```python
from build123d import *

# Parameters (mm, degrees)
SKETCH1_R           = 38.1
BOSS_EXTRUDE1_DEPTH = 4.826
SKETCH2_R           = 38.1
BOSS_EXTRUDE2_DEPTH = 3.302
BOSS_EXTRUDE2_DRAFT = -70
SKETCH3_R           = 47.172170439
BOSS_EXTRUDE3_DEPTH = 3.81
SKETCH4_R           = 46.472170439
CUT_EXTRUDE1_DEPTH  = 0.2
SKETCH6_R           = 34.772170439
SKETCH6_R_2         = 12.7
CUT_EXTRUDE2_DEPTH  = 2.7
SKETCH8_R           = 12.7
BOSS_EXTRUDE4_DEPTH = 50.8
SKETCH10_R          = 7.35
CUT_EXTRUDE5_DEPTH  = 3
SKETCH13_R          = 6.4
CUT_EXTRUDE9_DEPTH  = 92.577748235
SKETCH15_R          = 37.5
BOSS_EXTRUDE6_DEPTH = 8
CUT_EXTRUDE10_REACH = 99.233
SKETCH16_R          = 2
SKETCH16_R_2        = 5.35
SKETCH17_R          = 20.71
SKETCH17_R_2        = 19.21
CUT_EXTRUDE11_DEPTH = 3


with BuildPart() as part:
    # Sketch1 → Boss-Extrude1 (new body)
    with BuildSketch(Plane(origin=(0, 0, 0), x_dir=(1, 0, 0), z_dir=(0, 1, 0))):
        with Locations(Location((0, 0, 0), (0, 0, 270))):
            Circle(SKETCH1_R)
    extrude(amount=BOSS_EXTRUDE1_DEPTH)


with BuildPart() as boss_extrude2_tool:
    # Sketch2 → Boss-Extrude2 (with draft: the straight prism first)
    with BuildSketch(Plane(origin=(0, 4.826, 0), x_dir=(1, 0, 0), z_dir=(0, 1, 0))):
        with Locations(Location((0, 0, 0), (0, 0, 270))):
            Circle(SKETCH2_R)
    extrude(amount=BOSS_EXTRUDE2_DEPTH)
    # Boss-Extrude2: the draft: its side faces are tilted about the plane it starts from
    boss_extrude2_sides = [boss_extrude2_tool.faces().sort_by_distance(p)[0] for p in [
        (0, 6.477, -38.1),
    ]]
    draft(boss_extrude2_sides, Plane(origin=(0, 4.826, 0), x_dir=(1, 0, 0), z_dir=(0, 1, 0)), BOSS_EXTRUDE2_DRAFT)


with BuildPart() as part_1:
    add(part.part)

    # Boss-Extrude2: add boss_extrude2_tool
    add(boss_extrude2_tool.part)

    # Sketch3 → Boss-Extrude3 (add)
    with BuildSketch(Plane(origin=(0, 8.128, 0), x_dir=(1, 0, 0), z_dir=(0, 1, 0))):
        with Locations(Location((0, 0, 0), (0, 0, 90))):
            Circle(SKETCH3_R)
    extrude(amount=BOSS_EXTRUDE3_DEPTH)

    # Sketch4 → Cut-Extrude1 (cut)
    with BuildSketch(Plane(origin=(0, 11.938, 0), x_dir=(1, 0, 0), z_dir=(0, 1, 0))):
        with Locations(Location((0, 0, 0), (0, 0, 270))):
            Circle(SKETCH4_R)
    extrude(amount=-CUT_EXTRUDE1_DEPTH, mode=Mode.SUBTRACT)

    # Sketch6 → Cut-Extrude2 (cut)
    with BuildSketch(Plane(origin=(0, 11.738, 0), x_dir=(1, 0, 0), z_dir=(0, 1, 0))):
        with Locations(Location((0, 0, 0), (0, 0, 270))):
            Circle(SKETCH6_R)
        with Locations(Location((0, 0, 0), (0, 0, 270))):
            Circle(SKETCH6_R_2, mode=Mode.SUBTRACT)
    extrude(amount=-CUT_EXTRUDE2_DEPTH, mode=Mode.SUBTRACT)

    # Sketch8 → Boss-Extrude4 (add)
    with BuildSketch(Plane.XZ):
        with Locations(Location((0, 0, 0), (0, 0, 90))):
            Circle(SKETCH8_R)
    extrude(amount=BOSS_EXTRUDE4_DEPTH)

    # Sketch10 → Cut-Extrude5 (cut)
    with BuildSketch(Plane(origin=(0, 11.738, 0), x_dir=(1, 0, 0), z_dir=(0, 1, 0))):
        with Locations(Location((0, 0, 0), (0, 0, 270))):
            Circle(SKETCH10_R)
    extrude(amount=-CUT_EXTRUDE5_DEPTH, mode=Mode.SUBTRACT)

    # Sketch13 → Cut-Extrude9 (cut, through all)
    with BuildSketch(Plane(origin=(0, -50.8, 0), x_dir=(-1, 0, 0), z_dir=(0, -1, 0))):
        with Locations(Location((0, 0, 0), (0, 0, 90))):
            Circle(SKETCH13_R)
    extrude(amount=-CUT_EXTRUDE9_DEPTH, mode=Mode.SUBTRACT)

    # Sketch15 → Boss-Extrude6 (add)
    with BuildSketch(Plane.XZ.offset(50.8)):
        with Locations(Location((0, 0, 0), (0, 0, 270))):
            Circle(SKETCH15_R)
    extrude(amount=BOSS_EXTRUDE6_DEPTH)

    # Sketch16 → Cut-Extrude10 (cut, up to next)
    with BuildSketch(Plane.XZ.offset(58.8), mode=Mode.PRIVATE) as cut_extrude10_sk1:
        with Locations(Location((0, 33.75, 0), (0, 0, 270))):
            Circle(SKETCH16_R)
    cut_extrude10_tool1 = extrude(cut_extrude10_sk1.sketch, amount=-CUT_EXTRUDE10_REACH, mode=Mode.PRIVATE) & part_1.part
    # Sketch16 → Cut-Extrude10 (cut, up to next)
    with BuildSketch(Plane.XZ.offset(58.8), mode=Mode.PRIVATE) as cut_extrude10_sk2:
        with Locations(Location((23.864853865, 23.864853865, 0), (0, 0, 270))):
            Circle(SKETCH16_R)
    cut_extrude10_tool2 = extrude(cut_extrude10_sk2.sketch, amount=-CUT_EXTRUDE10_REACH, mode=Mode.PRIVATE) & part_1.part
    # Sketch16 → Cut-Extrude10 (cut, up to next)
    with BuildSketch(Plane.XZ.offset(58.8), mode=Mode.PRIVATE) as cut_extrude10_sk3:
        with Locations(Location((33.75, 0, 0), (0, 0, 270))):
            Circle(SKETCH16_R)
    cut_extrude10_tool3 = extrude(cut_extrude10_sk3.sketch, amount=-CUT_EXTRUDE10_REACH, mode=Mode.PRIVATE) & part_1.part
    # Sketch16 → Cut-Extrude10 (cut, up to next)
    with BuildSketch(Plane.XZ.offset(58.8), mode=Mode.PRIVATE) as cut_extrude10_sk4:
        with Locations(Location((23.864853865, -23.864853865, 0), (0, 0, 270))):
            Circle(SKETCH16_R)
    cut_extrude10_tool4 = extrude(cut_extrude10_sk4.sketch, amount=-CUT_EXTRUDE10_REACH, mode=Mode.PRIVATE) & part_1.part
    # Sketch16 → Cut-Extrude10 (cut, up to next)
    with BuildSketch(Plane.XZ.offset(58.8), mode=Mode.PRIVATE) as cut_extrude10_sk5:
        with Locations(Location((0, -33.75, 0), (0, 0, 270))):
            Circle(SKETCH16_R)
    cut_extrude10_tool5 = extrude(cut_extrude10_sk5.sketch, amount=-CUT_EXTRUDE10_REACH, mode=Mode.PRIVATE) & part_1.part
    # Sketch16 → Cut-Extrude10 (cut, up to next)
    with BuildSketch(Plane.XZ.offset(58.8), mode=Mode.PRIVATE) as cut_extrude10_sk6:
        with Locations(Location((-23.864853865, -23.864853865, 0), (0, 0, 270))):
            Circle(SKETCH16_R)
    cut_extrude10_tool6 = extrude(cut_extrude10_sk6.sketch, amount=-CUT_EXTRUDE10_REACH, mode=Mode.PRIVATE) & part_1.part
    # Sketch16 → Cut-Extrude10 (cut, up to next)
    with BuildSketch(Plane.XZ.offset(58.8), mode=Mode.PRIVATE) as cut_extrude10_sk7:
        with Locations(Location((-33.75, 0, 0), (0, 0, 270))):
            Circle(SKETCH16_R)
    cut_extrude10_tool7 = extrude(cut_extrude10_sk7.sketch, amount=-CUT_EXTRUDE10_REACH, mode=Mode.PRIVATE) & part_1.part
    # Sketch16 → Cut-Extrude10 (cut, up to next)
    with BuildSketch(Plane.XZ.offset(58.8), mode=Mode.PRIVATE) as cut_extrude10_sk8:
        with Locations(Location((-23.864853865, 23.864853865, 0), (0, 0, 270))):
            Circle(SKETCH16_R)
    cut_extrude10_tool8 = extrude(cut_extrude10_sk8.sketch, amount=-CUT_EXTRUDE10_REACH, mode=Mode.PRIVATE) & part_1.part
    # Sketch16 → Cut-Extrude10 (cut, up to next)
    with BuildSketch(Plane.XZ.offset(58.8), mode=Mode.PRIVATE) as cut_extrude10_sk9:
        with Locations(Location((0, 0, 0), (0, 0, 270))):
            Circle(SKETCH16_R_2)
    cut_extrude10_tool9 = extrude(cut_extrude10_sk9.sketch, amount=-CUT_EXTRUDE10_REACH, mode=Mode.PRIVATE) & part_1.part
    add(cut_extrude10_tool1.solids().sort_by_distance((0, -58.8, 33.75))[0], mode=Mode.SUBTRACT)
    add(cut_extrude10_tool2.solids().sort_by_distance((23.864854, -58.8, 23.864854))[0], mode=Mode.SUBTRACT)
    add(cut_extrude10_tool3.solids().sort_by_distance((33.75, -58.8, 0))[0], mode=Mode.SUBTRACT)
    add(cut_extrude10_tool4.solids().sort_by_distance((23.864854, -58.8, -23.864854))[0], mode=Mode.SUBTRACT)
    add(cut_extrude10_tool5.solids().sort_by_distance((0, -58.8, -33.75))[0], mode=Mode.SUBTRACT)
    add(cut_extrude10_tool6.solids().sort_by_distance((-23.864854, -58.8, -23.864854))[0], mode=Mode.SUBTRACT)
    add(cut_extrude10_tool7.solids().sort_by_distance((-33.75, -58.8, 0))[0], mode=Mode.SUBTRACT)
    add(cut_extrude10_tool8.solids().sort_by_distance((-23.864854, -58.8, 23.864854))[0], mode=Mode.SUBTRACT)
    add(cut_extrude10_tool9.solids().sort_by_distance((0, -58.8, 0))[0], mode=Mode.SUBTRACT)

    # Sketch17 → Cut-Extrude11 (cut)
    with BuildSketch(Plane.XZ.offset(58.8)):
        with Locations(Location((0, 0, 0), (0, 0, 270))):
            Circle(SKETCH17_R)
        with Locations(Location((0, 0, 0), (0, 0, 270))):
            Circle(SKETCH17_R_2, mode=Mode.SUBTRACT)
    extrude(amount=-CUT_EXTRUDE11_DEPTH, mode=Mode.SUBTRACT)


solid = part_1.part
```
Input: part model. Units: mm. Frame: model coordinates. A direction names the side the tool comes from. Round coordinates to 2 decimals unless told otherwise and drop trailing zeros. Loops run counter-clockwise (first coordinate to the right, second up) from the corner with the lowest first, then second, coordinate; pieces in that order, holes last. Notation, with made-up numbers: M 19,14.25 L 66,14.25 A30 ccw 66,40.25 Z; hole C -17,-29 d7. An arc over 180 degrees is marked long. Answer in a Markdown table with one row per item. Add a question column.
1. Section A-A (y = -52.5). Give the number of separate pieces and of enclosed holes in the cut face, and give its area (3 significant figures).
2. Contact query for flat-ended pins moving along their axis: pin 1 (3 mm diameter, centred on x = -23.86, z = 23.86, fed in from +Y); pin 2 (10 mm diameter, centred on y = -44, z = -16.5, fed in from +X); pin 3 (2.5 mm diameter, centred on x = 23.86, z = -23.86, fed in from -Y). Output: stop coordinate, or through.
3. Ray query, probe 1 along Y at (x, z) = (11.5, 8); probe 2 along X at (y, z) = (10, 0); probe 3 along X at (y, z) = (-5.5, -5) (3 decimals). Return the intervals inside material, ascending.
4. Set-up query: faces 1 (the face through (7, 8.738, 1)), 2 (the face through (35, 11.938, -31)), 3 (the face through (-14, -55.8, -14)), 4 (the face through (-16, -50.8, 1)). Return all of +Z, -Z, +X, -X, +Y, -Y with unobstructed straight access to the full face (end or side cutting, diameter ignored); none if empty.
5. Mould query, pull axis X, two halves, no side actions, for faces 5 (the face through (-7.7, 10.4, -10.1)), 6 (the face through (7.7, -25, -10.1)), 7 (the face through (1, 0, 16)). Classes: released by +X, released by -X, zero draft, split by the parting line, or undercut.
6. Section D-D (y = -43). Output: boundary loops of the cut face in (x, z).
Values follow:
| question | item | result |
|---|---|---|
| 1 | separate pieces | 1 |
| 1 | enclosed holes | 9 |
| 1 | area | 4,230 mm^2 |
| 2 | pin 1 | y = 11.74 |
| 2 | pin 2 | x = 5.39 |
| 2 | pin 3 | y = 0 |
| 3 | probe 1 | -58.8 to -50.8, 0 to 9.04 |
| 3 | probe 2 | -47.17 to -34.77, -12.7 to -7.35, 7.35 to 12.7, 34.77 to 47.17 |
| 3 | probe 3 | -11.674 to -3.995, 3.995 to 11.674 |
| 4 | face 1 | +Y |
| 4 | face 2 | +Z, -Z, +X, -X, +Y |
| 4 | face 3 | -Y |
| 4 | face 4 | none |
| 5 | face 5 | undercut |
| 5 | face 6 | split by the parting line |
| 5 | face 7 | zero draft |
| 6 | outline | C 0,0 d25.4; hole C 0,0 d12.8 |
